Could you check a few things on this model? Use its own coordinates, in mm. Face numbers are marked on the shaded views. Round coordinates to 2 decimals unless told otherwise and drop trailing zeros. Loops run counter-clockwise (first coordinate to the right, second up) from the corner with the lowest first, then second, coordinate; pieces in that order, holes last. Notation, with made-up numbers: (-3.75, 74.5) -> (17.25, 74.5) arc R25 ccw to (17.25, 106.5) -> close; hole circle Ø5 at (16, -23). An arc over 180 degrees is marked (long way). One line per item, written item: value.
Autodesk Inventor part; units mm, degrees
ref_plane "NUT_XY" through (0, 0, 0) normal (0, 0, 1) x (1, 0, 0)
ref_plane "NUT_YZ" through (0, 0, 0) normal (1, 0, 0) x (0, 1, 0)
ref_plane "NUT_ZX" through (0, 0, 0) normal (0, 1, 0) x (0, 0, 1)
sketch "Sketch_8" plane through (0, 0, 0) normal (1, 0, 0) x (0, 1, 0)
  line L0 (0, -2.794) -> (0, 0)
  line L1 (0, 0) -> (3.8989, 0)
  line L2 (3.8989, 0) -> (4.6787, -0.2089)
  line L3 (4.6787, -0.2089) -> (4.6787, -2.5851)
  line L4 (4.6787, -2.5851) -> (3.8989, -2.794)
  line L5 (3.8989, -2.794) -> (0, -2.794)
  line L6 (0, -2.794) -> (0, 0)
sketch "Sketch_10" plane through (0, 0, 0) normal (0, 0, 1) x (1, 0, 0)
  line L0 (-7.7978, 7.7978) -> (-7.7978, -7.7978)
  line L1 (-7.7978, -7.7978) -> (7.7978, -7.7978)
  line L2 (7.7978, -7.7978) -> (7.7978, 7.7978)
  line L3 (7.7978, 7.7978) -> (-7.7978, 7.7978)
  line L4 (-3.8989, 2.251) -> (-3.8989, -2.251)
  line L5 (-3.8989, -2.251) -> (0, -4.5021)
  line L6 (0, -4.5021) -> (3.8989, -2.251)
  line L7 (3.8989, -2.251) -> (3.8989, 2.251)
  line L8 (3.8989, 2.251) -> (0, 4.5021)
  line L9 (0, 4.5021) -> (-3.8989, 2.251)
revolve "Revolution1" add sketch "Sketch_8" angle 360 about axis through (0, 0, -2.794) along (0, 0, -1)
extrude "Extrusion1" cut sketch "Sketch_10" against normal blind 2.794
sketch "Sketch_13" plane through (0, 0, 0) normal (1, 0, 0) x (0, 1, 0)
  line L0 (0, -2.794) -> (0, 0)
  line L1 (0, 0) -> (1.5875, 0)
  line L2 (1.5875, 0) -> (1.2433, -0.3442)
  line L3 (1.2433, -0.3442) -> (1.2433, -2.4498)
  line L4 (1.2433, -2.4498) -> (1.5875, -2.794)
  line L5 (1.5875, -2.794) -> (0, -2.794)
  line L6 (0, -2.794) -> (0, 0)
revolve "Revolution2" cut sketch "Sketch_13" angle 360 about axis through (0, 0, -2.794) along (0, 0, -1)
thread "Thread1"
ref_plane "NUT_XY" through (0, 0, 0) normal (0, 0, 1) x (1, 0, 0)
ref_plane "NUT_YZ" through (0, 0, 0) normal (1, 0, 0) x (0, 1, 0)
ref_plane "NUT_ZX" through (0, 0, 0) normal (0, 1, 0) x (0, 0, 1)
ref_plane "a1_XY" through (-3.8989, 3.8989, 0) normal (0, 0, 1) x (1, 0, 0)
ref_plane "a1_YZ" through (-3.8989, 3.8989, 0) normal (1, 0, 0) x (0, 1, 0)
ref_plane "a1_ZX" through (-3.8989, 3.8989, 0) normal (0, 1, 0) x (0, 0, 1)
ref_plane "a2_XY" through (3.8989, 3.8989, 0) normal (0, 0, 1) x (1, 0, 0)
ref_plane "a2_YZ" through (3.8989, 3.8989, 0) normal (1, 0, 0) x (0, 1, 0)
ref_plane "a2_ZX" through (3.8989, 3.8989, 0) normal (0, 1, 0) x (0, 0, 1)
ref_plane "b1_XY" through (0, 3.8989, 0) normal (1, 0, 0) x (0, 0, -1)
ref_plane "b1_YZ" through (0, 3.8989, 0) normal (0, 0, -1) x (0, 1, 0)
ref_plane "b1_ZX" through (0, 3.8989, 0) normal (0, 1, 0) x (1, 0, 0)
ref_plane "b2_XY" through (0, 3.8989, -2.794) normal (1, 0, 0) x (0, 0, -1)
ref_plane "b2_YZ" through (0, 3.8989, -2.794) normal (0, 0, -1) x (0, 1, 0)
ref_plane "b2_ZX" through (0, 3.8989, -2.794) normal (0, 1, 0) x (1, 0, 0)
ref_plane "e_XY" through (0, 0, -2.794) normal (1, 0, 0) x (0, 0, -1)
ref_plane "e_YZ" through (0, 0, -2.794) normal (0, 0, -1) x (0, 1, 0)
ref_plane "e_ZX" through (0, 0, -2.794) normal (0, 1, 0) x (1, 0, 0)
ref_plane "th1_XY" through (0, 1.5875, -2.794) normal (1, 0, 0) x (0, 0, -1)
ref_plane "th1_YZ" through (0, 1.5875, -2.794) normal (0, 0, -1) x (0, 1, 0)
ref_plane "th1_ZX" through (0, 1.5875, -2.794) normal (0, 1, 0) x (1, 0, 0)
ref_plane "th2_XY" through (0, -1.5875, -2.794) normal (1, 0, 0) x (0, 0, -1)
ref_plane "th2_YZ" through (0, -1.5875, -2.794) normal (0, 0, -1) x (0, 1, 0)
ref_plane "th2_ZX" through (0, -1.5875, -2.794) normal (0, 1, 0) x (1, 0, 0)
ref_plane "ol1_XY" through (0, 0, -3.8989) normal (0, 1, 0) x (1, 0, 0)
ref_plane "ol1_YZ" through (0, 0, -3.8989) normal (1, 0, 0) x (0, 0, -1)
ref_plane "ol1_ZX" through (0, 0, -3.8989) normal (0, 0, -1) x (0, 1, 0)
ref_plane "ol2_XY" through (2.794, 0, -3.8989) normal (0, 1, 0) x (1, 0, 0)
ref_plane "ol2_YZ" through (2.794, 0, -3.8989) normal (1, 0, 0) x (0, 0, -1)
ref_plane "ol2_ZX" through (2.794, 0, -3.8989) normal (0, 0, -1) x (0, 1, 0)
properties part number "D-3745"
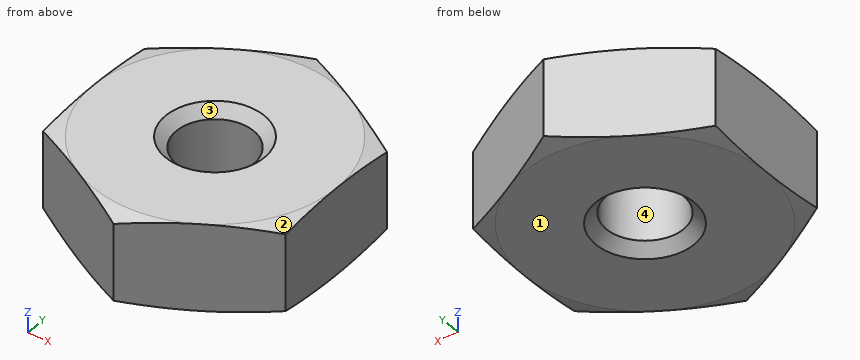
(1) We'd pull the mould along X, two halves only. Please class the marked faces 1, 2, 3 and 4: +X half, -X half, draft (parallel to the pull), parting line (faces both ways), or undercut.
Results below:
face 1: draft
face 2: +X half
face 3: undercut
face 4: undercut
(2) For pin 1 Ø1.5 at (x, z) = (2, -0.5) entering from -Y; pin 2 Ø2 at (x, y) = (0, 0) entering from +Z (1 decimal), each with a flat end and sliding along its axis, tell me the tip position at first contact or that it passes through.
Results below:
pin 1: stops at y = -3.78
pin 2: passes through
(3) Imagine slicing it at A-A on z = -2.35. Write out the boundary of the cut face in (x, y).
Results below:
outline: (-3.9, -2.25) -> (0, -4.5) -> (3.9, -2.25) -> (3.9, 2.25) -> (0, 4.5) -> (-3.9, 2.25) -> close; hole circle Ø2.49 at (0, 0)
(4) Please list where these lines run through material, in increasing order: L1, parallel to X at y = 0, z = -1.75; L2, parallel to X at y = 1, z = -2.25; L3, parallel to Y at x = 0.25, z = -2.3.
Results below:
L1: x = -3.9 to -1.24, 1.24 to 3.9
L2: x = -3.9 to -0.74, 0.74 to 3.9
L3: y = -4.36 to -1.22, 1.22 to 4.36
